```python
from build123d import *

# Parameters (mm, degrees)
CROQUIS1_R              = 4.5
CROQUIS1_R_2            = 3
SALIENTE_EXTRUIR1_DEPTH = 2
CROQUIS2_R              = 5.5
CROQUIS2_R_2            = 4
SALIENTE_EXTRUIR2_DEPTH = 3.2
REDONDEO1_R             = 2


with BuildPart() as part:
    # Croquis1 → Saliente-Extruir1 (new body)
    with BuildSketch(Plane.XY):
        Circle(CROQUIS1_R)
        Circle(CROQUIS1_R_2, mode=Mode.SUBTRACT)
    extrude(amount=SALIENTE_EXTRUIR1_DEPTH)

    # Croquis2 → Saliente-Extruir2 (add)
    with BuildSketch(Plane.XY.offset(2)):
        Circle(CROQUIS2_R)
        Circle(CROQUIS2_R_2, mode=Mode.SUBTRACT)
    extrude(amount=SALIENTE_EXTRUIR2_DEPTH)

    # Redondeo1
    # the kernel refuses this fillet: 2 mm, written as the material it adds along each edge
    with BuildSketch(Plane(origin=(0, 0, 2), x_dir=(1, 0, 0), z_dir=(0, -1, 0))) as redondeo1_piece_1:
        with BuildLine():
            CenterArc((6.5, -1.732050808), REDONDEO1_R, 120, 60)
            Line((5.5, 0), (5.48, 0.034641016))
            ThreePointArc((5.48, 0.034641016), (5, 0.04), (4.5, 0.04))
            Line((4.5, 0.04), (4.46, 0))
            Line((4.46, 0), (4.46, -1.732050808))
            Line((4.46, -1.732050808), (4.5, -1.732050808))
        make_face()
    revolve(axis=Axis((0, 0, 2), (0, 0, 1)))


solid = part.part
```
Could you check a few things on this model? Use its own coordinates, in mm. A direction names the side the tool comes from. Give positions to 0.01 mm unless a question says otherwise; leave off trailing zeros. Write each loop counter-clockwise with the first axis right and the second up, starting at its lowest first coordinate (ties: lowest second). Pieces come first, ordered by that corner, then holes. Notation, with made-up numbers: (79, 37) - (125, 37) arc R16 ccw to (125, 64) - close; hole circle Ø11 at (52.25, 33). An arc over 180 degrees is marked (long way). One line per item, written item: value. Start each with the question number.
Item 1: If we mould it in two halves opening along Y, with no side actions, what happens to faces 1 (the face through (-3, 0, 1)), 2 (the face through (-1.19, -5.37, 3.58)), 3 (the face through (1, -3, 0))? For each: +Y half, -Y half, draft (parallel to the pull), parting line (faces both ways), or undercut.
Item 2: Please list where these lines run through material, in increasing order: line 1 (Y direction, x = 0, z = 4.2); line 2 (X direction, y = -0.5, z = 0.75); line 3 (Y direction, x = -3.25, z = 4.25). Write a range as from..to.
Item 3: I'm going to push flat-ended pins straight in: pin 1 (1 mm diameter, centred on y = -3.5, z = 4, fed in from -X); pin 2 (1 mm diameter, centred on x = 2, y = -1, fed in from +Z); pin 3 (3 mm diameter, centred on y = -2, z = 2.5, fed in from +X); pin 4 (1 mm diameter, centred on x = -2.5, z = 4, fed in from -Y). Where does each tip first touch, or does it pass through?
Item 4: Imagine slicing it at D-D, the plane z = 0.9. List the corners of the cut face in (x, y) for me (1 decimal), and give its area (3 significant figures).
Item 5: Imagine slicing it at A-A, the plane x = 0. List the corners of the cut face in (y, z) for me, and give its area (3 significant figures).
Item 6: Which directions (+Z, -Z, +X, -X, +Y, -Y) give clear straight access to the entire face, cutting with the end or side of a thin tool? Please do faces 4 (the face through (-0.867, -3.905, 3.578)), 5 (the face through (-4, -2, 5.2)).
Item 7: Imagine slicing it at C-C, the plane z = 3.45. List the corners of the cut face in (x, y) for me.
Geometry says:
1. face 1: undercut
1. face 2: parting line
1. face 3: draft
2. line 1: -5.5..-4, 4..5.5
2. line 2: -4.53..-2.96, 2.96..4.53
2. line 3: -4.44..-2.33, 2.33..4.44
3. pin 1: x = -4.61
3. pin 2: through
3. pin 3: x = 5.48
3. pin 4: y = -5.12
4. outline: circle Ø9.2 at (0, 0); hole circle Ø6 at (0, 0)
4. area: 38.3 mm^2
5. outline: (-5.5, 2) arc R2 cw to (-4.5, 0.27) - (-4.5, 0) - (-3, 0) - (-3, 2) - (-4, 2) - (-4, 5.2) - (-5.5, 5.2) - close; (3, 0) - (4.5, 0) - (4.5, 0.27) arc R2 cw to (5.5, 2) - (5.5, 5.2) - (4, 5.2) - (4, 2) - (3, 2) - close
5. area: 16.6 mm^2
6. face 4: +Z
6. face 5: +Z, +X, -X, +Y, -Y
7. outline: circle Ø11 at (0, 0); hole circle Ø8 at (0, 0)
